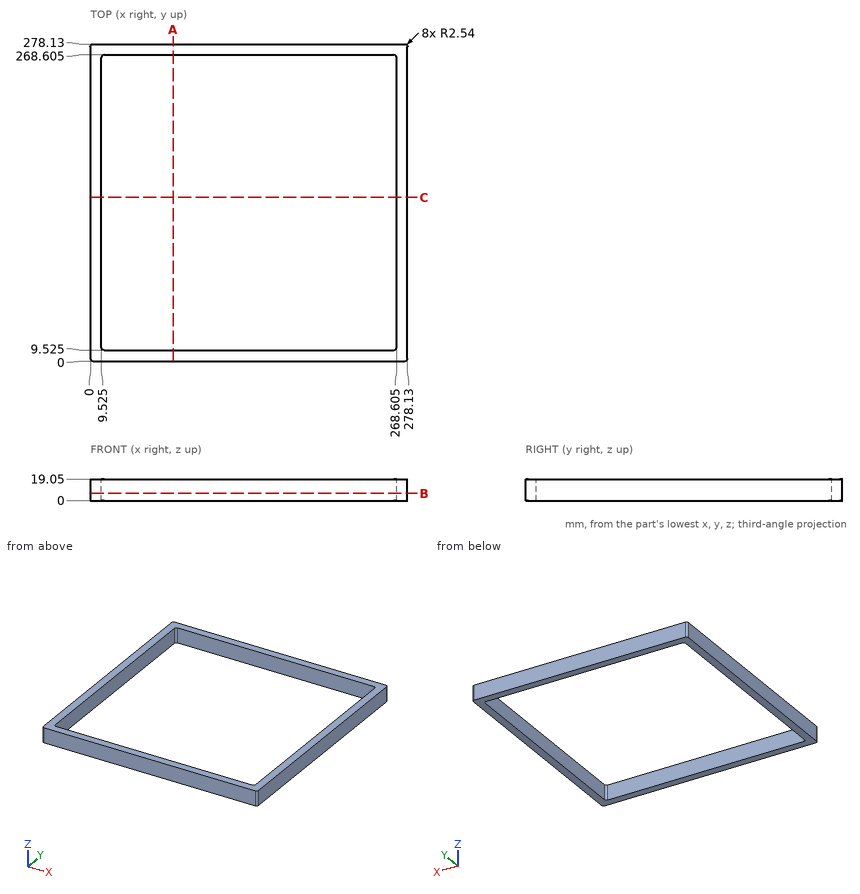
Can you work these out from the drawing? Everything is in mm from the part's minimum corner. Coordinates: 2 decimals unless noted, no trailing zeros. Loops run counter-clockwise (first coordinate to the right, second up) from the corner with the lowest first, then second, coordinate; pieces in that order, holes last.
1) Imagine slicing it at B-B (z = 6.5). List the corners of the cut face in (x, y) for me (3 decimals).
Reported:
outline: (0, 2.54) arc R2.54 ccw to (2.54, 0) - (275.59, 0) arc R2.54 ccw to (278.13, 2.54) - (278.13, 275.59) arc R2.54 ccw to (275.59, 278.13) - (2.54, 278.13) arc R2.54 ccw to (0, 275.59) - close; hole (9.525, 12.065) arc R2.54 ccw to (12.065, 9.525) - (266.065, 9.525) arc R2.54 ccw to (268.605, 12.065) - (268.605, 266.065) arc R2.54 ccw to (266.065, 268.605) - (12.065, 268.605) arc R2.54 ccw to (9.525, 266.065) - close
2) Please list where this line runs through material, in increasing order: line 1 along Y through (x, z) = (252, 11.5) (3 decimals).
Reported:
line 1: y = 0 to 9.525, 268.605 to 278.13
3) Imagine slicing it at A-A (x = 72.5). List the corners of the cut face in (y, z) for me (3 decimals), and give its area (3 significant figures).
Reported:
outline: (0, 0) - (9.525, 0) - (9.525, 19.05) - (0, 19.05) - close; (268.605, 0) - (278.13, 0) - (278.13, 19.05) - (268.605, 19.05) - close
area: 363 mm2
